Part print with two shaded views. Sizes in mm from the minimum x, y, z corner. Round coordinates to 2 decimals unless told otherwise and drop trailing zeros. Write each loop counter-clockwise with the first axis right and the second up, starting at its lowest first coordinate (ties: lowest second). Pieces come first, ordered by that corner, then holes. Notation, with made-up numbers: (4, 51) -> (62, 51) arc R18 ccw to (62, 56) -> close; hole circle Ø2 at (33.5, 81.25). An arc over 180 degrees is marked (long way). Return JSON: item names as keys, results as strings.
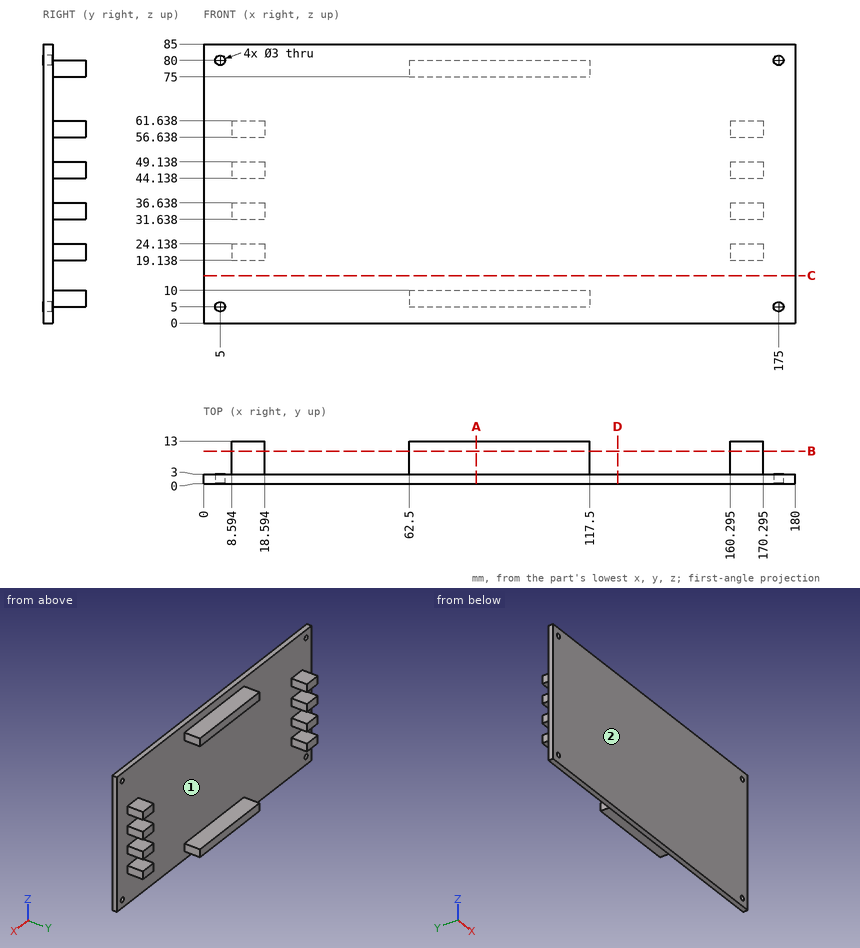
Q1. Pin check, flat tips, straight feed: pin 1 Ø5.5 at (y, z) = (10, 76.5) entering from +X; pin 2 Ø3 at (x, y) = (165.5, 7) entering from -Z; pin 3 Ø2.5 at (y, z) = (10, 58) entering from +X (3 decimals). Stop position of each tip, or through.
Verdict:
{"pin 1": "stops at x = 117.5", "pin 2": "stops at z = 19.14", "pin 3": "stops at x = 170.295"}
Q2. Two-plate mould, pull along Z, no slides. Class the marked faces 1 and 2: +Z half, -Z half, draft (parallel to the pull), parting line (faces both ways), or undercut.
Verdict:
{"face 1": "undercut", "face 2": "draft"}
Q3. Saw through at A-A on x = 83. List the corners of the cut face in (y, z).
Verdict:
{"outline": "(0, 0) -> (3, 0) -> (3, 5) -> (13, 5) -> (13, 10) -> (3, 10) -> (3, 75) -> (13, 75) -> (13, 80) -> (3, 80) -> (3, 85) -> (0, 85) -> close"}
Q4. Wall check: L1, parallel to X at y = 1.1, z = 80; L2, parallel to Z at x = 5, y = 0.8; L3, parallel to Z at x = 68, y = 7. Give the ranges that are in metal, low to high.
Verdict:
{"L1": "x = 0 to 3.5, 6.5 to 173.5, 176.5 to 180", "L2": "z = 0 to 3.5, 6.5 to 78.5, 81.5 to 85", "L3": "z = 5 to 10, 75 to 80"}
Q5. Saw through at D-D on x = 126. List the corners of the cut face in (y, z), then the cut area to 3 significant figures.
Verdict:
{"outline": "(0, 0) -> (3, 0) -> (3, 85) -> (0, 85) -> close", "area": "255 mm²"}
Q6. Saw through at C-C on z = 14.5. List the corners of the cut face in (x, y).
Verdict:
{"outline": "(0, 0) -> (180, 0) -> (180, 3) -> (0, 3) -> close"}
Q7. Saw through at B-B on y = 10. Count the separate pieces of the cut face and the enclosed holes in it, then the cut area to 3 significant figures.
Verdict:
{"separate pieces": "10", "enclosed holes": "0", "area": "950 mm²"}
